The model under review builds one solid part; all positions refer to its coordinate system, in mm. Coordinates: 2 decimals unless noted, no trailing zeros. Loops run counter-clockwise (first coordinate to the right, second up) from the corner with the lowest first, then second, coordinate; pieces in that order, holes last. Notation, with made-up numbers: (33, -36) - (48, -36) arc R10 cw to (48, -26) - close; hole circle Ø10 at (74, 27.25). An arc over 180 degrees is marked (long way). Answer in a Markdown table with one row per item. Add a question column.
(1) We need section A-A on x = 73.5. Write out the cut boundary in (y, z).
(2) For P1, Ø5, axis at y = 126, z = 9, coming from the +X side; P2, Ø5.5, axis at x = -12.5, z = 12.5, coming from the +Y side; P3, Ø5.5, axis at y = 162.5, z = 9.5, coming from the -X side, all flat-tipped, find the tip position at first contact; note any pin that passes through.
(3) For line 1 along Y through (x, z) = (-35.5, 4.5); line 2 along X through (y, z) = (150.5, 11.5); line 3 along Y through (x, z) = (161.5, 14), list the stretches that pass through material, from the lowest coordinate up.
from build123d import *

# Parameters (mm, degrees)
F0_W      = 400
F0_H      = 350
F1_DEPTH  = 19
F3_DEPTH  = 19.001
F5_DEPTH  = 19.0010001
F7_DEPTH  = 19.0010001
F9_DEPTH  = 19.0010001
F10_W     = 152.0328149199
F10_H     = 37.6462221146
F11_DEPTH = 19.0010001


with BuildPart() as f1:
    # F0 (on Top) → F1 (new body)
    with BuildSketch(Plane.XY):
        Rectangle(F0_W, F0_H)
    extrude(amount=F1_DEPTH)

    # F2 (on face) → F3 (cut, through all)
    with BuildSketch(Plane.XY.offset(19)):
        with BuildLine():
            Line((200, 175), (151.3424734159, 175))
            add(Edge.make_bspline(
                [(151.3424734159, 175), (163.628163973, 174.5270389431), (195.7541165045, 169.8113391239), (199.6478987114, 135.2669980399), (200, 122.4896438138)],
                knots=[0.1722762022, 0.1722762022, 0.1722762022, 0.1722762022, 0.4977126924, 0.8513762401, 0.8513762401, 0.8513762401, 0.8513762401], degree=3))
            Line((200, 122.4896438138), (200, 175))
        make_face()
    extrude(amount=-F3_DEPTH, mode=Mode.SUBTRACT)

    # F4 (on face) → F5 (cut, through all)
    with BuildSketch(Plane.XY.offset(19)):
        with BuildLine():
            add(Edge.make_bspline(
                [(-140.7613994596, 175), (-150.110855442, 173.3851097158), (-195.0889612855, 174.4196814068), (-199.6708864934, 136.6798470352), (-200, 127.4311682667)],
                knots=[0, 0, 0, 0, 0.4272708141, 0.7095152118, 0.7095152118, 0.7095152118, 0.7095152118], degree=3))
            Line((-140.7613994596, 175), (-200, 175))
            Line((-200, 175), (-200, 127.4311682667))
        make_face()
    extrude(amount=-F5_DEPTH, mode=Mode.SUBTRACT)

    # F6 (on face) → F7 (cut, through all)
    with BuildSketch(Plane.XY.offset(19)):
        with BuildLine():
            add(Edge.make_bspline(
                [(-200, -100.9678691626), (-198.025562325, -115.9679433742), (-200.7344906485, -168.6506935141), (-154.2425532874, -174.1251325706), (-143.251940608, -175)],
                knots=[0, 0, 0, 0, 0.432032055, 0.8175239829, 0.8175239829, 0.8175239829, 0.8175239829], degree=3))
            Line((-200, -100.9678691626), (-200, -175))
            Line((-200, -175), (-143.251940608, -175))
        make_face()
    extrude(amount=-F7_DEPTH, mode=Mode.SUBTRACT)

    # F8 (on face) → F9 (cut, through all)
    with BuildSketch(Plane.XY.offset(19)):
        with BuildLine():
            add(Edge.make_bspline(
                [(131.8723261356, -175), (147.6494681392, -172.9795732693), (191.3520223086, -173.7383685692), (199.6154264724, -111.8109622903), (200, -111.4782392979)],
                knots=[0, 0, 0, 0, 0.4868319345, 0.9480551396, 0.9480551396, 0.9480551396, 0.9480551396], degree=3))
            Line((131.8723261356, -175), (200, -175))
            Line((200, -175), (200, -112.0964959264))
            Line((200, -112.0964959264), (200, -111.4782392979))
        make_face()
    extrude(amount=-F9_DEPTH, mode=Mode.SUBTRACT)

    # F10 (on face) → F11 (cut, through all)
    with BuildSketch(Plane.XY.offset(19)):
        with Locations((4.6131424606, 156.1768889427)):
            Rectangle(F10_W, F10_H)
    extrude(amount=-F11_DEPTH, mode=Mode.SUBTRACT)


solid = f1.part
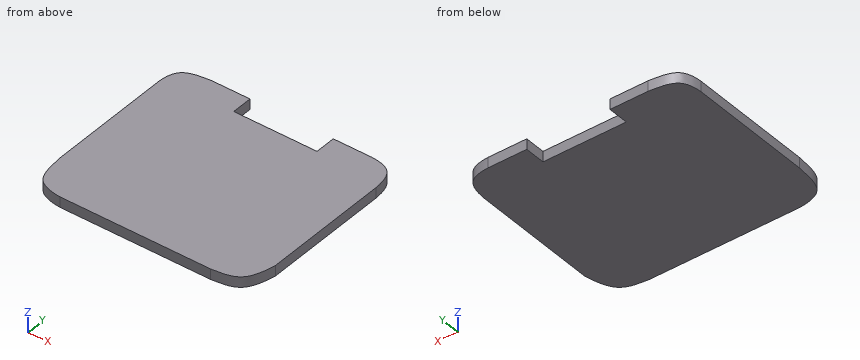
Outcome:
| question | item | result |
|---|---|---|
| 1 | outline | (-175, 0) - (137.35, 0) - (137.35, 19) - (-175, 19) - close |
| 2 | P1 | x = 199.97 |
| 2 | P2 | y = 137.35 |
| 2 | P3 | x = -190.36 |
| 3 | line 1 | -175 to 137.35 |
| 3 | line 2 | -195.74 to -71.4, 80.63 to 195.5 |
| 3 | line 3 | -170.64 to 174.16 |
